Model file for the job. Use its own axes, mm. Face numbers are marked on the shaded views. A direction names the side the tool comes from. Round coordinates to 2 decimals unless told otherwise and drop trailing zeros. Loops run counter-clockwise (first coordinate to the right, second up) from the corner with the lowest first, then second, coordinate; pieces in that order, holes last. Notation, with made-up numbers: (84, 74.5) -> (140, 74.5) arc R33 ccw to (140, 108.5) -> close; hole circle Ø4 at (63, 5.5). An arc over 180 degrees is marked (long way). Use a Markdown table: item, result. Add a question column.
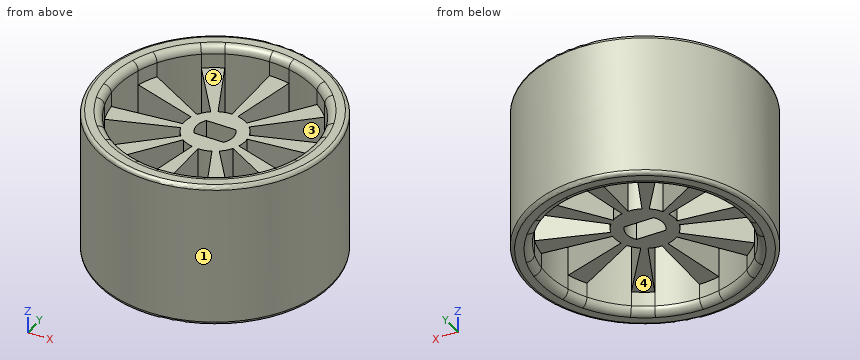
```python
from build123d import *
from build123d.topology import SkipClean

# Parameters (mm, degrees)
SKETCH1_R           = 16
BOSS_EXTRUDE1_DEPTH = 20
CUT_EXTRUDE1_DEPTH  = 20
CUT_EXTRUDE2_DEPTH  = 20
SKETCH5_R           = 13.379368239
CUT_EXTRUDE4_DEPTH  = 3
CUT_EXTRUDE5_START  = -3
SKETCH6_R           = 13.379368239
CUT_EXTRUDE5_DEPTH  = 3
FILLET1_R           = 1
FILLET2_R           = 0.5


with BuildPart() as part:
    # Sketch1 → Boss-Extrude1 (new body)
    with BuildSketch(Plane.XY):
        Circle(SKETCH1_R)
    extrude(amount=BOSS_EXTRUDE1_DEPTH)

    # Sketch3 → Cut-Extrude1 (cut)
    with BuildSketch(Plane.XY):
        with BuildLine():
            Line((-2, 1.5), (2, 1.5))
            ThreePointArc((2, 1.5), (2.5, 0), (2, -1.5))
            Line((2, -1.5), (-2, -1.5))
            ThreePointArc((-2, -1.5), (-2.5, 0), (-2, 1.5))
        make_face()
    extrude(amount=CUT_EXTRUDE1_DEPTH, mode=Mode.SUBTRACT)

    # Sketch4 → Cut-Extrude2 (cut)
    with BuildSketch(Plane.XY):
        with BuildLine():
            Line((3.955700901, -1.285285135), (12.724535348, -4.13445216))
            ThreePointArc((12.724535348, -4.13445216), (13.30607466, -1.398524802), (13.30607466, 1.398524802))
            Line((13.30607466, 1.398524802), (4.136485151, 0.434762108))
            ThreePointArc((4.136485151, 0.434762108), (4.136485151, -0.434762108), (3.955700901, -1.285285135))
        make_face()
        with BuildLine():
            Line((3.090940028, 2.783094902), (9.942808275, 8.952544783))
            ThreePointArc((9.942808275, 8.952544783), (11.586872782, 6.68968412), (12.724535348, 4.13445216))
            Line((12.724535348, 4.13445216), (3.955700901, 1.285285135))
            ThreePointArc((3.955700901, 1.285285135), (3.602033539, 2.079635034), (3.090940028, 2.783094902))
        make_face()
        with BuildLine():
            Line((2.444757606, -3.364920169), (7.864195336, -10.82413628))
            ThreePointArc((7.864195336, -10.82413628), (9.942808275, -8.952544783), (11.586872782, -6.68968412))
            Line((11.586872782, -6.68968412), (3.602033539, -2.079635034))
            ThreePointArc((3.602033539, -2.079635034), (3.090940028, -2.783094902), (2.444757606, -3.364920169))
        make_face()
        with BuildLine():
            Line((0, -4.159270067), (0, -13.379368239))
            ThreePointArc((0, -13.379368239), (2.781727073, -13.086996943), (5.441879324, -12.222661081))
            Line((5.441879324, -12.222661081), (1.691727545, -3.799682277))
            ThreePointArc((1.691727545, -3.799682277), (0.864760872, -4.068380037), (0, -4.159270067))
        make_face()
        with BuildLine():
            Line((-2.444757606, -3.364920169), (-7.864195336, -10.82413628))
            ThreePointArc((-7.864195336, -10.82413628), (-5.441879324, -12.222661081), (-2.781727073, -13.086996943))
            Line((-2.781727073, -13.086996943), (-0.864760872, -4.068380037))
            ThreePointArc((-0.864760872, -4.068380037), (-1.691727545, -3.799682277), (-2.444757606, -3.364920169))
        make_face()
        with BuildLine():
            Line((-3.955700901, -1.285285135), (-12.724535348, -4.13445216))
            ThreePointArc((-12.724535348, -4.13445216), (-11.586872782, -6.68968412), (-9.942808275, -8.952544783))
            Line((-9.942808275, -8.952544783), (-3.090940028, -2.783094902))
            ThreePointArc((-3.090940028, -2.783094902), (-3.602033539, -2.079635034), (-3.955700901, -1.285285135))
        make_face()
        with BuildLine():
            Line((-3.955700901, 1.285285135), (-12.724535348, 4.13445216))
            ThreePointArc((-12.724535348, 4.13445216), (-13.30607466, 1.398524802), (-13.30607466, -1.398524802))
            Line((-13.30607466, -1.398524802), (-4.136485151, -0.434762108))
            ThreePointArc((-4.136485151, -0.434762108), (-4.136485151, 0.434762108), (-3.955700901, 1.285285135))
        make_face()
        with BuildLine():
            Line((-2.444757606, 3.364920169), (-7.864195336, 10.82413628))
            ThreePointArc((-7.864195336, 10.82413628), (-9.942808275, 8.952544783), (-11.586872782, 6.68968412))
            Line((-11.586872782, 6.68968412), (-3.602033539, 2.079635034))
            ThreePointArc((-3.602033539, 2.079635034), (-3.090940028, 2.783094902), (-2.444757606, 3.364920169))
        make_face()
        with BuildLine():
            Line((0, 4.159270067), (0, 13.379368239))
            ThreePointArc((0, 13.379368239), (-2.781727073, 13.086996943), (-5.441879324, 12.222661081))
            Line((-5.441879324, 12.222661081), (-1.691727545, 3.799682277))
            ThreePointArc((-1.691727545, 3.799682277), (-0.864760872, 4.068380037), (0, 4.159270067))
        make_face()
        with BuildLine():
            Line((2.444757606, 3.364920169), (7.864195336, 10.82413628))
            ThreePointArc((7.864195336, 10.82413628), (5.441879324, 12.222661081), (2.781727073, 13.086996943))
            Line((2.781727073, 13.086996943), (0.864760872, 4.068380037))
            ThreePointArc((0.864760872, 4.068380037), (1.691727545, 3.799682277), (2.444757606, 3.364920169))
        make_face()
    extrude(amount=CUT_EXTRUDE2_DEPTH, mode=Mode.SUBTRACT)

    # Sketch5 → Cut-Extrude4 (cut)
    with SkipClean():  # the faces are left unmerged after this step: merging them gives an invalid solid
        with BuildSketch(Plane.XY):
            with Locations(Location((0, 0, 0), (0, 0, 186))):
                Circle(SKETCH5_R)
        extrude(amount=CUT_EXTRUDE4_DEPTH, mode=Mode.SUBTRACT)

    # Sketch6 → Cut-Extrude5 (cut)
    with SkipClean():  # the faces are left unmerged after this step: merging them gives an invalid solid
        with BuildSketch(Plane.XY.offset(20).offset(CUT_EXTRUDE5_START)):
            Circle(SKETCH6_R)
        extrude(amount=CUT_EXTRUDE5_DEPTH, mode=Mode.SUBTRACT)

    # Fillet1
    fillet1_edges = [part.edges().sort_by_distance(p)[0] for p in [
        (13.30607466, -1.398524802, 0),
        (13.214646015, -2.092994313, 20),
    ]]
    fillet(fillet1_edges, radius=FILLET1_R)

    # Fillet2
    fillet2_edges = [part.edges().sort_by_distance(p)[0] for p in [
        (-16, 0, 0),
        (-16, 0, 20),
    ]]
    fillet(fillet2_edges, radius=FILLET2_R)


solid = part.part
```
1) Tool access for the marked faces 3 and 4: list every direction of +Z, -Z, +X, -X, +Y, -Y with a clear straight run to the whole face (end or side of a thin tool).
2) Pin check, flat tips, straight feed: pin 1 Ø2 at (x, z) = (7, 15) entering from -Y; pin 2 Ø2 at (y, z) = (5.5, 10) entering from +X; pin 3 Ø2 at (y, z) = (11, 6) entering from -X. Stop position of each tip, or through.
3) Cut at B-B on z = 1.75. Write the cut outline in (x, y).
4) Pull direction Y, two halves, no side cores. Call the marked faces 1 and 2: +Y half, -Y half, draft (parallel to the pull), parting line (faces both ways), or undercut.
5) Cut at A-A on y = 0. Write the cut outline in (x, z), and give its area (3 significant figures).
6) Cut at C-C on z = 8.75. Count the separate pieces of the cut face and the enclosed holes in it, and give its area (3 significant figures).
7) Wall check: probe 1 along Y at (x, z) = (0.5, 11.25); probe 2 along X at (y, z) = (8.5, 12); probe 3 along X at (y, z) = (11.5, 13.5). Give the ranges that are in metal, low to high. Write a range as from..to.
Established:
| question | item | result |
|---|---|---|
| 1 | face 3 | +Z, -Z |
| 1 | face 4 | -Z |
| 2 | pin 1 | stops at y = -14.83 |
| 2 | pin 2 | stops at x = 15.35 |
| 2 | pin 3 | stops at x = -12.49 |
| 3 | outline | circle Ø32 at (0, 0); hole circle Ø26.76 at (0, 0) |
| 4 | face 1 | parting line |
| 4 | face 2 | undercut |
| 5 | outline | (-16, 0.5) arc R0.5 ccw to (-15.5, 0) -> (-14.38, 0) arc R1 ccw to (-13.38, 1) -> (-13.38, 19) arc R1 ccw to (-14.38, 20) -> (-15.5, 20) arc R0.5 ccw to (-16, 19.5) -> close; (-4.16, 3) -> (-2.5, 3) -> (-2.5, 17) -> (-4.16, 17) -> close; (2.5, 3) -> (4.16, 3) -> (4.16, 17) -> (2.5, 17) -> close; (13.38, 1) arc R1 ccw to (14.38, 0) -> (15.5, 0) arc R0.5 ccw to (16, 0.5) -> (16, 19.5) arc R0.5 ccw to (15.5, 20) -> (14.38, 20) arc R1 ccw to (13.38, 19) -> close |
| 5 | area | 150 mm^2 |
| 6 | separate pieces | 1 |
| 6 | enclosed holes | 11 |
| 6 | area | 452 mm^2 |
| 7 | probe 1 | y = -15.99..-13.37, -4.13..-1.5, 1.5..15.99 |
| 7 | probe 2 | x = -13.56..-10.33, -6.18..-3.78, 0..1.81, 6.18..9.44, 10.33..13.56 |
| 7 | probe 3 | x = -11.12..-5.12, 0..2.44, 6.84..11.12 |
